Design review of the part built by this model. Coordinates are the model's own, in mm. A direction names the side the tool comes from. Round coordinates to 2 decimals unless told otherwise and drop trailing zeros. Loops run counter-clockwise (first coordinate to the right, second up) from the corner with the lowest first, then second, coordinate; pieces in that order, holes last. Notation, with made-up numbers: (75.5, 7) - (117.5, 7) arc R28 ccw to (117.5, 46) - close; hole circle Ø11 at (-26.5, 57.5). An arc over 180 degrees is marked (long way). Answer as CSV lines item,"result". Start each with the question number.
(1) Consider section C-C (z = 17). Give the boundary of the cut face in (x, y), and give its area (3 significant figures).
(2) For P1, Ø3, axis at x = 9.5, y = 4, coming from the +Z side; P2, Ø8, axis at x = 32.5, z = 16.5, coming from the -Y side; P3, Ø8, axis at y = 2, z = 16, coming from the -X side, all flat-tipped, find the tip position at first contact; note any pin that passes through.
(3) For faces 1 (the flat face through (17, 1.5, 9)), 2 (the flat face through (29, -9.5, 10)), 3 (the flat face through (12, -6, 3)), 4 (the flat face through (20, -6.5, -2)), 5 (the flat face through (20, 11, 0)), list the 3-axis set-ups (+Z, -Z, +X, -X, +Y, -Y) from which the entire face can be reached by the end or side of a thin tool; tool diameter is ignored.
(4) Wall thickness on L1, parallel to Z at x = 32.5, y = 1.5; L2, parallel to Z at x = 4, y = -10.75; L3, parallel to Y at x = 27, z = -1.75: over which ranges is each line inside the solid? List them lowest first.
(5) Consider section B-B (x = 32.5). Give the boundary of the cut face in (y, z), and give its area (3 significant figures).
(6) Mouldability with a two-part tool opening along Y and no side actions: class faces 6 (the flat face through (20, 6.5, -2)), 7 (the flat face through (20, 12.5, -1)), 8 (the flat face through (20, -11, 0)), 9 (the flat face through (20, 0, 0)) as released by +Y, released by -Y, zero draft, split by the parting line, or undercut.
(7) Consider section A-A (y = 7.75). Give the boundary of the cut face in (x, z), and give its area (3 significant figures).
(8) Consider section D-D (y = 3). Give the boundary of the cut face in (x, z).
from build123d import *

# Parameters (mm, degrees)
F1_DEPTH = 40
F3_R     = 3.5
F4_DEPTH = 9.5
F5_DEPTH = 1.5


with BuildPart() as f1:
    # F0 (on Right) → F1 (new body)
    with BuildSketch(Plane.YZ):
        Polygon((-6.5, 0), (0, 0), (0, 3), (-9.5, 3), (-9.5, 0), (-12.5, 0), (-12.5, -3), (-6.5, -3), align=None)
    extrude(amount=F1_DEPTH)

    # F2: F1 across plane


with BuildPart() as f1_1:
    add(f1.part)
    add(f1.part.mirror(Plane.XZ))

    # F3 (on Front) → F4 (join, symmetric)
    with BuildSketch(Plane.XZ):
        with BuildLine():
            Line((25, 3), (40, 3))
            Line((40, 3), (40, 16.5))
            ThreePointArc((40, 16.5), (35.971113, 23.148412), (28.212967, 22.65397))
            ThreePointArc((28.212967, 22.65397), (25.851588, 19.971113), (25, 16.5))
            Line((25, 16.5), (25, 3))
        make_face()
        with Locations((32.5, 16.5)):
            Circle(F3_R, mode=Mode.SUBTRACT)
    extrude(amount=F4_DEPTH, both=True)

    # F3 (on Front) → F5 (join, symmetric)
    with BuildSketch(Plane.XZ):
        with BuildLine():
            Line((0, 3), (25, 3))
            Line((25, 3), (25, 16.5))
            ThreePointArc((25, 16.5), (25.851588, 19.971113), (28.212967, 22.65397))
            Line((28.212967, 22.65397), (0, 3))
        make_face()
    extrude(amount=F5_DEPTH, both=True)


solid = f1_1.part
Determined:
1,outline,"(20.1, -1.5) - (25.02, -1.5) - (25.02, -9.5) - (29.04, -9.5) - (29.04, 9.5) - (25.02, 9.5) - (25.02, 1.5) - (20.1, 1.5) - close; (35.96, -9.5) - (39.98, -9.5) - (39.98, 9.5) - (35.96, 9.5) - close"
1,area,"167 mm^2"
2,P1,"stops at z = 3"
2,P2,"stops at y = -9.5"
2,P3,"stops at x = 12.96"
3,face 1,"+Z, -X, +Y"
3,face 2,"+Z, +X, -X, -Y"
3,face 3,"+Z, -X, -Y"
3,face 4,"-Z, +X, -X"
3,face 5,"+Z, +X, -X, +Y"
4,L1,"z = 0 to 13, 20 to 24"
4,L2,"z = -3 to 0"
4,L3,"y = -12.5 to -6.5, 6.5 to 12.5"
5,outline,"(-12.5, -3) - (-6.5, -3) - (-6.5, 0) - (6.5, 0) - (6.5, -3) - (12.5, -3) - (12.5, 0) - (9.5, 0) - (9.5, 13) - (-9.5, 13) - (-9.5, 0) - (-12.5, 0) - close; (-9.5, 20) - (9.5, 20) - (9.5, 24) - (-9.5, 24) - close"
5,area,"359 mm^2"
6,face 6,"undercut"
6,face 7,"released by +Y"
6,face 8,"zero draft"
6,face 9,"undercut"
7,outline,"(0, -3) - (40, -3) - (40, 16.5) arc R7.5 ccw to (28.21, 22.65) arc R7.5 ccw to (25, 16.5) - (25, 3) - (0, 3) - close; hole circle Ø7 at (32.5, 16.5)"
7,area,"492 mm^2"
8,outline,"(0, 0) - (40, 0) - (40, 16.5) arc R7.5 ccw to (28.21, 22.65) arc R7.5 ccw to (25, 16.5) - (25, 3) - (0, 3) - close; hole circle Ø7 at (32.5, 16.5)"
